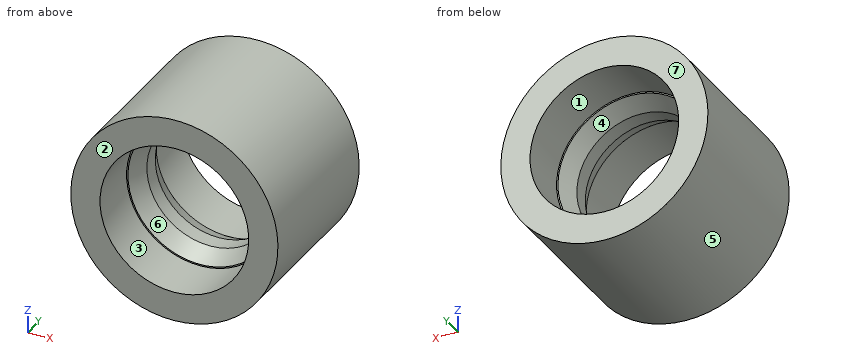
from build123d import *
from OCP.BRepFilletAPI import BRepFilletAPI_MakeChamfer

# Parameters (mm, degrees)
SKETCH1_R           = 12
SKETCH1_R_2         = 5
BOSS_EXTRUDE1_DEPTH = 15
SKETCH2_R           = 7
CUT_EXTRUDE1_DEPTH  = 5.1
CUT_EXTRUDE2_START  = -5.1
SKETCH3_R           = 7
CUT_EXTRUDE2_DEPTH  = 5.1
BOSS_EXTRUDE2_START = -4.8
SKETCH4_R           = 5
SKETCH4_R_2         = 3
BOSS_EXTRUDE2_DEPTH = 4.8
SKETCH5_R           = 17.644165846
SKETCH5_R_2         = 10
CUT_EXTRUDE3_DEPTH  = 17.1
SKETCH6_R           = 7.1
CUT_EXTRUDE4_DEPTH  = 5.1
CUT_EXTRUDE5_START  = -5.1
SKETCH7_R           = 7.1
CUT_EXTRUDE5_DEPTH  = 5.1
SKETCH8_R           = 14.835126002
SKETCH8_R_2         = 9.75
CUT_EXTRUDE7_DEPTH  = 26
SKETCH9_R           = 6.0214871
CUT_EXTRUDE8_DEPTH  = 10
BOSS_EXTRUDE3_START = 0.2
SKETCH10_R          = 7.1
SKETCH10_R_2        = 6.0214871
BOSS_EXTRUDE3_DEPTH = 0.2
SKETCH11_R          = 7.1
SKETCH11_R_2        = 6.0214871
BOSS_EXTRUDE4_DEPTH = 0.2
CHAMFER2_SIZE       = 0.85
CHAMFER2_SIZE2      = 1.822830882
BOSS_EXTRUDE5_REACH = 22.375
SKETCH12_R          = 9.75
SKETCH12_R_2        = 7


with BuildPart() as part:
    # Sketch1 → Boss-Extrude1 (new body)
    with BuildSketch(Plane(origin=(0, 0, 0), x_dir=(1, 0, 0), z_dir=(0, 1, 0))):
        with Locations(Location((0, 0, 0), (0, 0, 270))):
            Circle(SKETCH1_R)
        with Locations(Location((0, 0, 0), (0, 0, 270))):
            Circle(SKETCH1_R_2, mode=Mode.SUBTRACT)
    extrude(amount=BOSS_EXTRUDE1_DEPTH)

    # Sketch2 → Cut-Extrude1 (cut)
    with BuildSketch(Plane.XZ):
        with Locations(Location((0, 0, 0), (0, 0, 270))):
            Circle(SKETCH2_R)
    extrude(amount=-CUT_EXTRUDE1_DEPTH, mode=Mode.SUBTRACT)

    # Sketch3 → Cut-Extrude2 (cut)
    with BuildSketch(Plane(origin=(0, 15, 0), x_dir=(1, 0, 0), z_dir=(0, 1, 0)).offset(CUT_EXTRUDE2_START)):
        with Locations(Location((0, 0, 0), (0, 0, 90))):
            Circle(SKETCH3_R)
    extrude(amount=CUT_EXTRUDE2_DEPTH, mode=Mode.SUBTRACT)

    # Sketch4 → Boss-Extrude2 (add)
    with BuildSketch(Plane(origin=(0, 9.9, 0), x_dir=(1, 0, 0), z_dir=(0, 1, 0)).offset(BOSS_EXTRUDE2_START)):
        Circle(SKETCH4_R)
        with Locations(Location((0, 0, 0), (0, 0, 270))):
            Circle(SKETCH4_R_2, mode=Mode.SUBTRACT)
    extrude(amount=BOSS_EXTRUDE2_DEPTH)

    # Sketch5 → Cut-Extrude3 (cut)
    with BuildSketch(Plane.XZ):
        Circle(SKETCH5_R)
        with Locations(Location((0, 0, 0), (0, 0, 270))):
            Circle(SKETCH5_R_2, mode=Mode.SUBTRACT)
    extrude(amount=-CUT_EXTRUDE3_DEPTH, mode=Mode.SUBTRACT)

    # Sketch6 → Cut-Extrude4 (cut)
    with BuildSketch(Plane.XZ):
        with Locations(Location((0, 0, 0), (0, 0, 270))):
            Circle(SKETCH6_R)
    extrude(amount=-CUT_EXTRUDE4_DEPTH, mode=Mode.SUBTRACT)

    # Sketch7 → Cut-Extrude5 (cut)
    with BuildSketch(Plane(origin=(0, 15, 0), x_dir=(1, 0, 0), z_dir=(0, 1, 0)).offset(CUT_EXTRUDE5_START)):
        with Locations(Location((0, 0, 0), (0, 0, 90))):
            Circle(SKETCH7_R)
    extrude(amount=CUT_EXTRUDE5_DEPTH, mode=Mode.SUBTRACT)

    # Sketch8 → Cut-Extrude7 (cut)
    with BuildSketch(Plane.XZ):
        Circle(SKETCH8_R)
        with Locations(Location((0, 0, 0), (0, 0, 270))):
            Circle(SKETCH8_R_2, mode=Mode.SUBTRACT)
    extrude(amount=-CUT_EXTRUDE7_DEPTH, mode=Mode.SUBTRACT)

    # Sketch9 → Cut-Extrude8 (cut)
    with BuildSketch(Plane(origin=(0, 9.9, 0), x_dir=(1, 0, 0), z_dir=(0, 1, 0))):
        with Locations(Location((0, 0, 0), (0, 0, 270))):
            Circle(SKETCH9_R)
    extrude(amount=-CUT_EXTRUDE8_DEPTH, mode=Mode.SUBTRACT)

    # Sketch10 → Boss-Extrude3 (add)
    with BuildSketch(Plane.XZ.offset(-5.1).offset(BOSS_EXTRUDE3_START)):
        with Locations(Location((0, 0, 0), (0, 0, 270))):
            Circle(SKETCH10_R)
        with Locations(Location((0, 0, 0), (0, 0, 90))):
            Circle(SKETCH10_R_2, mode=Mode.SUBTRACT)
    extrude(amount=-BOSS_EXTRUDE3_DEPTH)

    # Sketch11 → Boss-Extrude4 (add)
    with BuildSketch(Plane(origin=(0, 9.9, 0), x_dir=(1, 0, 0), z_dir=(0, 1, 0))):
        with Locations(Location((0, 0, 0), (0, 0, 90))):
            Circle(SKETCH11_R)
        with Locations(Location((0, 0, 0), (0, 0, 270))):
            Circle(SKETCH11_R_2, mode=Mode.SUBTRACT)
    extrude(amount=BOSS_EXTRUDE4_DEPTH)

    # Chamfer2: one chamfer whose edges measure the first distance from different faces: ONE call of the kernel's chamfer builder (chamfer() names one face for all edges)
    chamfer2_edges_1 = [part.edges().sort_by_distance(p)[0] for p in [
        (0, 4.9, -6.0214871),
    ]]
    chamfer2_side_1 = [part.faces().sort_by_distance(p)[0] for p in [
        (0, 4.9, 6.899181674),
    ]]
    chamfer2_edges_2 = [part.edges().sort_by_distance(p)[0] for p in [
        (0, 10.1, -6.0214871),
    ]]
    chamfer2_side_2 = [part.faces().sort_by_distance(p)[0] for p in [
        (0, 10.1, 6.899181674),
    ]]
    chamfer2 = BRepFilletAPI_MakeChamfer(part.part.solid().wrapped)
    for e in chamfer2_edges_1:
        chamfer2.Add(CHAMFER2_SIZE, CHAMFER2_SIZE2, e.wrapped, chamfer2_side_1[0].wrapped)  # the first distance lies on this face
    for e in chamfer2_edges_2:
        chamfer2.Add(CHAMFER2_SIZE, CHAMFER2_SIZE2, e.wrapped, chamfer2_side_2[0].wrapped)  # the first distance lies on this face
    add(Compound.cast(chamfer2.Shape()), mode=Mode.REPLACE)

    # Boss-Extrude5: up to this face of the body (flat: up to its plane)
    boss_extrude5_end = Plane(part.part.faces().sort_by_distance((0, 0, 9.474228355))[0])
    # Sketch12 → Boss-Extrude5 (add, up to the picked face)
    with BuildSketch(Plane(origin=(0, 15, 0), x_dir=(1, 0, 0), z_dir=(0, 1, 0)), mode=Mode.PRIVATE) as boss_extrude5_sk1:
        with Locations(Location((0, 0, 0), (0, 0, 90))):
            Circle(SKETCH12_R)
        with Locations(Location((0, 0, 0), (0, 0, 270))):
            Circle(SKETCH12_R_2, mode=Mode.SUBTRACT)
    boss_extrude5_tool1 = split(extrude(boss_extrude5_sk1.sketch, amount=-BOSS_EXTRUDE5_REACH, mode=Mode.PRIVATE), bisect_by=boss_extrude5_end, keep=Keep.BOTH, mode=Mode.PRIVATE)
    add(boss_extrude5_tool1.solids().sort_by(Axis((0, 15, 9.474228), (0, -1, 0)))[0])


solid = part.part
Could you check a few things on this model? Use its own coordinates, in mm. Face numbers are marked on the shaded views. A direction names the side the tool comes from. Give positions to 0.01 mm unless a question says otherwise; leave off trailing zeros. Order: outer loops, then holes, each group sorted by start corner. A loop starts at its lowest first (then second) coordinate and runs counter-clockwise, first axis right, second up. Notation, with made-up numbers: (53.5, 2) - (85.5, 2) arc R15 ccw to (85.5, 8) - close; hole circle Ø6 at (55.5, -36). An arc over 180 degrees is marked (long way). One line per question, with ' | ' between items. Start each with the question number.
Item 1: Thinking about a two-plate mould opening in Z: for the marked faces 4, 5, 6 and 7, which applies, pulls with the +Z half, pulls with the -Z half, needs draft (parallel to the pull), parting line crosses it, or undercut?
Item 2: I want a section at C-C on y = 7.5. Write out the boundary of the cut face in (x, z), then the cut area to 3 significant figures.
Item 3: I want a section at B-B on x = 0. Write out the boundary of the cut face in (y, z).
Item 4: I want a section at D-D on z = -8. Write out the boundary of the cut face in (x, y), then the cut area to 3 significant figures.
Item 5: I want a section at A-A on z = 0. Write out the boundary of the cut face in (x, y), then the cut area to 3 significant figures.
Item 6: For the marked faces 1, 2 and 3, which set-ups out of +Z, -Z, +X, -X, +Y, -Y let a thin tool reach every point of the face, with its end or its side?
Item 7: I need wall thicknesses on probe 1 along X at (y, z) = (12.15, 0); probe 2 along X at (y, z) = (7.8, 0); probe 3 along Z at (x, y) = (-5.5, 5.5). Which ranges of each line are inside material? Lowest first, please. Write a range as [from, to].
Item 8: I'm going to push flat-ended pins straight in: pin 1 Ø2 at (x, y) = (6, 4) entering from -Z; pin 2 Ø1.5 at (x, y) = (1.5, 1.5) entering from +Z; pin 3 Ø8 at (y, z) = (10, 6.5) entering from +X. Where does each tip first touch, or does it pass through?
Verdict:
1) face 4: undercut | face 5: parting line crosses it | face 6: undercut | face 7: needs draft
2) outline: circle Ø19.5 at (0, 0); hole circle Ø12.04 at (0, 0) | area: 185 mm^2
3) outline: (0, -9.75) - (15, -9.75) - (15, -7) - (10.1, -7) - (10.1, -6.87) - (8.28, -6.02) - (6.72, -6.02) - (4.9, -6.87) - (4.9, -7) - (0, -7) - close; (0, 7) - (4.9, 7) - (4.9, 6.87) - (6.72, 6.02) - (8.28, 6.02) - (10.1, 6.87) - (10.1, 7) - (15, 7) - (15, 9.75) - (0, 9.75) - close
4) outline: (-5.57, 0) - (5.57, 0) - (5.57, 15) - (-5.57, 15) - close | area: 167 mm^2
5) outline: (-9.75, 0) - (-7, 0) - (-7, 4.9) - (-6.87, 4.9) - (-6.02, 6.72) - (-6.02, 8.28) - (-6.87, 10.1) - (-7, 10.1) - (-7, 15) - (-9.75, 15) - close; (6.02, 6.72) - (6.87, 4.9) - (7, 4.9) - (7, 0) - (9.75, 0) - (9.75, 15) - (7, 15) - (7, 10.1) - (6.87, 10.1) - (6.02, 8.28) - close | area: 89.6 mm^2
6) face 1: +Y | face 2: +Z, -Z, +X, -X, -Y | face 3: -Y
7) probe 1: [-9.75, -7], [7, 9.75] | probe 2: [-9.75, -6.02], [6.02, 9.75] | probe 3: [-8.05, -3.63], [3.63, 8.05]
8) pin 1: z = -8.37 | pin 2: z = 9.72 | pin 3: x = 9.42
